Build history of the part. All positions in model axes, mm. A direction names the side the tool comes from. Round coordinates to 2 decimals unless told otherwise and drop trailing zeros. Loops run counter-clockwise (first coordinate to the right, second up) from the corner with the lowest first, then second, coordinate; pieces in that order, holes last. Notation, with made-up numbers: (31, 84) - (59, 84) arc R13 ccw to (59, 105) - close; hole circle Ø5 at (-7, -25.5). An arc over 180 degrees is marked (long way). Put each result on its own line as item: value. Start each with the question number.
from build123d import *

# Parameters (mm, degrees)
SKETCH1_W           = 44.8
SKETCH1_H           = 72
SKETCH1_R           = 1.55
BOSS_EXTRUDE1_DEPTH = 2
CHAMFER2_SIZE       = 0.2
FILLET3_R           = 3


with BuildPart() as part:
    # Sketch1 → Boss-Extrude1 (new body)
    with BuildSketch(Plane(origin=(0, 0, 0), x_dir=(1, 0, 0), z_dir=(0, 1, 0))):
        Rectangle(SKETCH1_W, SKETCH1_H)
        with Locations((-16.6, -33.25)):
            Circle(SKETCH1_R, mode=Mode.SUBTRACT)
        with Locations((1.4, -33.25)):
            Circle(SKETCH1_R, mode=Mode.SUBTRACT)
        with Locations((19.4, -33.25)):
            Circle(SKETCH1_R, mode=Mode.SUBTRACT)
        with Locations((-16.6, 33.25)):
            Circle(SKETCH1_R, mode=Mode.SUBTRACT)
        with Locations((1.4, 33.25)):
            Circle(SKETCH1_R, mode=Mode.SUBTRACT)
        with Locations((19.4, 33.25)):
            Circle(SKETCH1_R, mode=Mode.SUBTRACT)
        with BuildLine():
            Line((17.3, -22.25), (-16.6, -22.25))
            ThreePointArc((-16.6, -22.25), (-17.519238816, -21.869238816), (-17.9, -20.95))
            Line((-17.9, -20.95), (-17.9, 20.95))
            ThreePointArc((-17.9, 20.95), (-17.519238816, 21.869238816), (-16.6, 22.25))
            Line((-16.6, 22.25), (17.3, 22.25))
            ThreePointArc((17.3, 22.25), (18.219238816, 21.869238816), (18.6, 20.95))
            Line((18.6, 20.95), (18.6, -20.95))
            ThreePointArc((18.6, -20.95), (18.219238816, -21.869238816), (17.3, -22.25))
        make_face(mode=Mode.SUBTRACT)
    extrude(amount=BOSS_EXTRUDE1_DEPTH)

    # Chamfer2
    chamfer2_edges = [part.edges().sort_by_distance(p)[0] for p in [
        (22.4, 1, -36),
        (22.4, 1, 36),
    ]]
    chamfer(chamfer2_edges, length=CHAMFER2_SIZE)

    # Fillet3
    fillet3_edges = [part.edges().sort_by_distance(p)[0] for p in [
        (-22.4, 1, 36),
        (-22.4, 1, -36),
    ]]
    fillet(fillet3_edges, radius=FILLET3_R)


solid = part.part
Item 1: Slice it at D-D (y = 0.85). Give the cut face in (x, z), plus the area to 3 significant figures.
Item 2: Slice it at C-C (x = 19.4). Give the cut face in (y, z), plus the area to 3 significant figures.
Item 3: Which spindle directions (+Z, -Z, +X, -X, +Y, -Y) get a long thin tool onto all of the face, cutting with end or side? Do faces 4 (the flat face through (-20, 2, -1)), 5 (the flat face through (18.6, 1, 0)). Say none if no direction does.
Item 4: Slice it at B-B (z = -4.5). Give the cut face in (x, y).
Item 5: Drop a flat-ended pin along its axis: pin 1 Ø5 at (x, z) = (19.4, -33.25) entering from -Y. Give the stop position or say it passes through.
Item 6: Slice it at A-A (x = 10.5). Give the cut face in (y, z).
Item 7: Drill centre lines: probe 1 along Z at (x, y) = (19.4, 1.15); probe 2 along X at (y, z) = (1.2, 33.25); probe 3 along Z at (x, y) = (1.5, 1.85). Where is each one in solid material? Low to high. Write a range as [from, to].
Item 8: Two-plate mould, pull along X, no slides. Class faces 1 (the flat face through (0, 1, -22.25)), 2 (the flat face through (1, 1, 36)), 3 (the flat face through (-22.4, 1, 0)): pulls with the +X half, pulls with the -X half, needs draft (parallel to the pull), parting line crosses it, or undercut.
Computed values:
1. outline: (-22.4, -33) arc R3 ccw to (-19.4, -36) - (22.2, -36) - (22.4, -35.8) - (22.4, 35.8) - (22.2, 36) - (-19.4, 36) arc R3 ccw to (-22.4, 33) - close; hole circle Ø3.1 at (-16.6, -33.25); hole circle Ø3.1 at (-16.6, 33.25); hole (-17.9, -20.95) arc R1.3 ccw to (-16.6, -22.25) - (17.3, -22.25) arc R1.3 ccw to (18.6, -20.95) - (18.6, 20.95) arc R1.3 ccw to (17.3, 22.25) - (-16.6, 22.25) arc R1.3 ccw to (-17.9, 20.95) - close; hole circle Ø3.1 at (1.4, -33.25); hole circle Ø3.1 at (1.4, 33.25); hole circle Ø3.1 at (19.4, -33.25); hole circle Ø3.1 at (19.4, 33.25)
1. area: 1,550 mm^2
2. outline: (0, -36) - (2, -36) - (2, -34.8) - (0, -34.8) - close; (0, -31.7) - (2, -31.7) - (2, 31.7) - (0, 31.7) - close; (0, 34.8) - (2, 34.8) - (2, 36) - (0, 36) - close
2. area: 132 mm^2
3. face 4: +Z, -Z, +X, -X, +Y
3. face 5: +Y, -Y
4. outline: (-22.4, 0) - (-17.9, 0) - (-17.9, 2) - (-22.4, 2) - close; (18.6, 0) - (22.4, 0) - (22.4, 2) - (18.6, 2) - close
5. pin 1: stops at y = 0
6. outline: (0, -36) - (2, -36) - (2, -22.25) - (0, -22.25) - close; (0, 22.25) - (2, 22.25) - (2, 36) - (0, 36) - close
7. probe 1: z = [-36, -34.8], [-31.7, 31.7], [34.8, 36]
7. probe 2: x = [-22.39, -18.15], [-15.05, -0.15], [2.95, 17.85], [20.95, 22.4]
7. probe 3: z = [-36, -34.8], [-31.7, -22.25], [22.25, 31.7], [34.8, 36]
8. face 1: undercut
8. face 2: needs draft
8. face 3: pulls with the -X half
